```python
from build123d import *

# Parameters (mm, degrees)
BOSS_EXTRUDE1_DEPTH = 110
SKETCH3_W           = 20.839202169
SKETCH3_H           = 50
SKETCH3_H_2         = 40.4
CUT_EXTRUDE1_DEPTH  = 110


with BuildPart() as part:
    # Sketch1 → Boss-Extrude1 (new body)
    with BuildSketch(Plane(origin=(0, 0, 0), x_dir=(1, 0, 0), z_dir=(0, 1, 0))):
        with BuildLine():
            ThreePointArc((-55, 0), (0, 55), (55, 0))
            Line((55, 0), (55, 10))
            Line((55, 10), (59.160797831, 10))
            ThreePointArc((59.160797831, 10), (0, 60), (-59.160797831, 10))
            Line((-59.160797831, 10), (-55, 10))
            Line((-55, 10), (-55, 0))
        make_face()
        with BuildLine():
            Line((-60, 0), (-55, 0))
            Line((-55, 0), (-55, 10))
            Line((-55, 10), (-59.160797831, 10))
            ThreePointArc((-59.160797831, 10), (-59.789831367, 5.017575617), (-60, 0))
        make_face()
        with BuildLine():
            ThreePointArc((-60, 0), (-59.789831367, 5.017575617), (-59.160797831, 10))
            Line((-59.160797831, 10), (-80, 10))
            Line((-80, 10), (-80, 0))
            Line((-80, 0), (-60, 0))
        make_face()
        with BuildLine():
            Line((60, 0), (80, 0))
            Line((80, 0), (80, 10))
            Line((80, 10), (59.160797831, 10))
            ThreePointArc((59.160797831, 10), (59.789831367, 5.017575617), (60, 0))
        make_face()
        with BuildLine():
            Line((55, 0), (60, 0))
            ThreePointArc((60, 0), (59.789831367, 5.017575617), (59.160797831, 10))
            Line((59.160797831, 10), (55, 10))
            Line((55, 10), (55, 0))
        make_face()
    extrude(amount=BOSS_EXTRUDE1_DEPTH)

    # Sketch3 → Cut-Extrude1 (cut)
    with BuildSketch(Plane(origin=(0, 0, -10), x_dir=(-1, 0, 0), z_dir=(0, 0, -1))):
        with Locations((-69.580398915, 34.8)):
            Rectangle(SKETCH3_W, SKETCH3_H)
        with Locations((69.580398915, 34.8)):
            Rectangle(SKETCH3_W, SKETCH3_H)
        with Locations((-69.580398915, 89.8)):
            Rectangle(SKETCH3_W, SKETCH3_H_2)
        with Locations((69.580398915, 89.8)):
            Rectangle(SKETCH3_W, SKETCH3_H_2)
    extrude(amount=-CUT_EXTRUDE1_DEPTH, mode=Mode.SUBTRACT)


solid = part.part
```
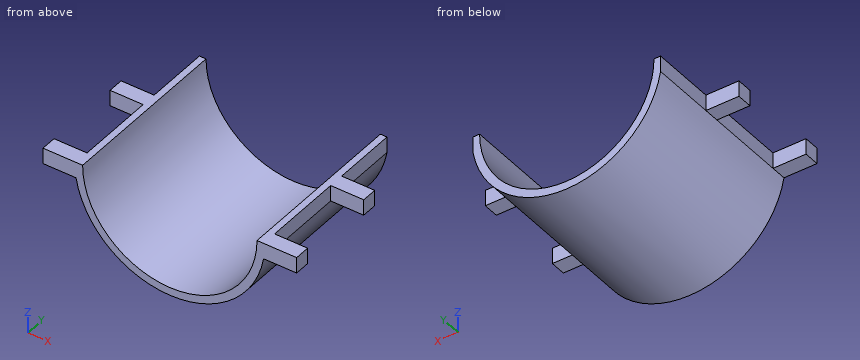
The listing builds one solid part. Answer for the finished solid, in the listing's coordinates (mm). Coordinates: 2 decimals unless noted, no trailing zeros. Write each loop counter-clockwise with the first axis right and the second up, starting at its lowest first coordinate (ties: lowest second). Pieces come first, ordered by that corner, then holes. Notation, with made-up numbers: M -25.5,23.25 L -8.5,23.25 A12 cw -8.5,32.25 Z; hole C 7.5,43.5 d2. An arc over 180 degrees is marked long. Use a Markdown table: item, result. Add a question column.
1. Section A-A (x = -70) is taken. Give the vertices of the cut face in (y, z), plus the area to 3 significant figures.
2. Straight lines are drawn through the part: line 1 along Z through (x, y) = (-0.5, 99.5); line 2 along X through (y, z) = (73, -24.5); line 3 along X through (y, z) = (46.5, -14). For each, find the intervals that lie inside material, in ascending order. Write a range as [from, to].
3. Section D-D (x = 1) is taken. Give the vertices of the cut face in (y, z), plus the area to 3 significant figures.
4. Given P1, Ø10, axis at y = 50, z = -21, coming from the +X side; P2, Ø2, axis at y = 59, z = -17.5, coming from the -X side; P3, Ø3, axis at x = -68.5, z = -4, coming from the +Y side, each flat-ended and moving along its own axis, determine where each tip first touches the part or whether it passes through.
5. Section C-C (z = -23.5) is taken. Give the vertices of the cut face in (x, y), plus the area to 3 significant figures.
6. Section B-B (y = 98) is taken. Give the vertices of the cut face in (x, z).
Data:
| question | item | result |
|---|---|---|
| 1 | outline | M 0,-10 L 9.8,-10 L 9.8,0 L 0,0 Z; M 59.8,-10 L 69.6,-10 L 69.6,0 L 59.8,0 Z |
| 1 | area | 196 mm2 |
| 2 | line 1 | z = [-60, -55] |
| 2 | line 2 | x = [-54.77, -49.24], [49.24, 54.77] |
| 2 | line 3 | x = [-58.34, -53.19], [53.19, 58.34] |
| 3 | outline | M 0,-59.99 L 110,-59.99 L 110,-54.99 L 0,-54.99 Z |
| 3 | area | 550 mm2 |
| 4 | P1 | stops at x = 57.83 |
| 4 | P2 | stops at x = -57.69 |
| 4 | P3 | stops at y = 69.6 |
| 5 | outline | M -55.21,0 L -49.73,0 L -49.73,110 L -55.21,110 Z; M 49.73,0 L 55.21,0 L 55.21,110 L 49.73,110 Z |
| 5 | area | 1,210 mm2 |
| 6 | outline | M -59.16,-10 A60 ccw 59.16,-10 L 59.16,0 L 55,0 A55 cw -55,0 L -59.16,0 Z |
